Work out the finished part from the listing and answer in its coordinate system (mm). Round coordinates to 2 decimals unless told otherwise and drop trailing zeros. Write each loop counter-clockwise with the first axis right and the second up, starting at its lowest first coordinate (ties: lowest second). Pieces come first, ordered by that corner, then holes. Notation, with made-up numbers: M 44,30 L 103,30 A15 ccw 103,58 Z; hole C 48.5,51 d5. An arc over 180 degrees is marked long. Answer in a Markdown table with one row per item.
```python
from build123d import *

# Parameters (mm, degrees)
SKETCH1_R          = 8.255
EXTRUDE1_DEPTH     = 6.096
SKETCH2_R          = 0.5
EXTRUDE2_DEPTH     = 3.429
FILLET1_R          = 1
SKETCH3_R          = 0.635
CUT_EXTRUDE1_DEPTH = 2.54
CIRPATTERN1_COUNT  = 4


with BuildPart() as part:
    # Sketch1 → Extrude1 (new, symmetric)
    with BuildSketch(Plane.XY):
        with Locations(Location((0, 0, 0), (0, 0, 180))):
            Circle(SKETCH1_R)
    extrude(amount=EXTRUDE1_DEPTH, both=True)

    # Sketch2 → Extrude2 (add)
    with BuildSketch(Plane(origin=(0, 0, -6.096), x_dir=(-1, 0, 0), z_dir=(0, 0, -1))):
        with Locations(Location((0, 5, 0), (0, 0, 180))):
            Circle(SKETCH2_R)
    extrude2 = extrude(amount=EXTRUDE2_DEPTH)

    # Mirror1: Extrude2 across plane
    add(extrude2.mirror(Plane.ZX))

    # Fillet1
    fillet1_edges = [part.edges().sort_by_distance(p)[0] for p in [
        (8.255, 0, 6.096),
    ]]
    fillet(fillet1_edges, radius=FILLET1_R)

    # Sketch3 → Cut-Extrude1 (cut)
    with BuildSketch(Plane.XY.offset(6.096)):
        Circle(SKETCH3_R)
        with BuildLine():
            ThreePointArc((3.388468085, 4.443425259), (3.922460813, 4.515354158), (3.850531915, 5.049346886))
            ThreePointArc((3.850531915, 5.049346886), (0, 6.35), (-3.850531915, 5.049346886))
            ThreePointArc((-3.850531915, 5.049346886), (-3.922460813, 4.515354158), (-3.388468085, 4.443425259))
            ThreePointArc((-3.388468085, 4.443425259), (0, 5.588), (3.388468085, 4.443425259))
        make_face()
        with BuildLine():
            ThreePointArc((3.741234039, 0.720602434), (4.187417686, 0.418539274), (4.489480846, 0.864722921))
            ThreePointArc((4.489480846, 0.864722921), (3.232892204, 3.232892204), (0.864722921, 4.489480846))
            ThreePointArc((0.864722921, 4.489480846), (0.418539274, 4.187417686), (0.720602434, 3.741234039))
            ThreePointArc((0.720602434, 3.741234039), (2.694076836, 2.694076836), (3.741234039, 0.720602434))
        make_face()
        with BuildLine():
            ThreePointArc((1.069473684, 1.727787614), (1.593960178, 1.851221476), (1.470526316, 2.375707969))
            ThreePointArc((1.470526316, 2.375707969), (0, 2.794), (-1.470526316, 2.375707969))
            ThreePointArc((-1.470526316, 2.375707969), (-1.593960178, 1.851221476), (-1.069473684, 1.727787614))
            ThreePointArc((-1.069473684, 1.727787614), (0, 2.032), (1.069473684, 1.727787614))
        make_face()
    cut_extrude1 = extrude(amount=-CUT_EXTRUDE1_DEPTH, mode=Mode.SUBTRACT)

    # CirPattern1: Cut-Extrude1 ×4 about axis
    cirpattern1_axis = Axis((0, 0, 0), (0, 0, 1))
    for i in range(1, CIRPATTERN1_COUNT):
        add(cut_extrude1.rotate(cirpattern1_axis, i * 360 / CIRPATTERN1_COUNT), mode=Mode.SUBTRACT)


solid = part.part
```
1. Determine the mould class of faces 1 (the flat face through (0, -5, -9.525)), 2 (the cylindrical face through (-0.065, -4.504, -7.786)) for opening direction Y: released by +Y, released by -Y, zero draft, split by the parting line, or undercut.
Calculated:
| item | result |
|---|---|
| face 1 | zero draft |
| face 2 | undercut |
2. The part is cut by section A-A (z = -6.75). Determine the outline of the cut face in (x, y), plus the area to 3 significant figures.
Calculated:
| item | result |
|---|---|
| outline | C 0,-5 d1; C 0,5 d1 |
| area | 1.57 mm² |
3. Given pin 1 (1.5 mm diameter, centred on x = 2, z = -6, fed in from -Y); pin 2 (1.5 mm diameter, centred on y = 6, z = -2.5, fed in from +X); pin 3 (6 mm diameter, centred on y = -3.5, z = -1.5, fed in from +X), each flat-ended and moving along its own axis, determine where each tip first touches the part or whether it passes through.
Calculated:
| item | result |
|---|---|
| pin 1 | stops at y = -8.16 |
| pin 2 | stops at x = 6.37 |
| pin 3 | stops at x = 8.24 |
4. Consider line 1 along Z through (x, y) = (-1.75, -1.25); line 2 along Y through (x, z) = (-2.25, 5.5) (3 decimals); line 3 along Z through (x, y) = (-6.25, -3). Determine where each line is inside the solid, lowest interval first. Write a range as from..to.
Calculated:
| item | result |
|---|---|
| line 1 | z = -6.1..3.56 |
| line 2 | y = -7.854..-5.938, -5.115..-3.98, -3.075..-1.595, 1.595..3.075, 3.98..5.115, 5.938..7.854 |
| line 3 | z = -6.1..6.1 |
5. The part is cut by section B-B (z = 1.5). Determine the outline of the cut face in (x, y) (3 decimals).
Calculated:
| item | result |
|---|---|
| outline | C 0,0 d16.51 |
